CAD build for the part. Positions are in the model's coordinates, mm. A direction names the side the tool comes from. Round coordinates to 2 decimals unless told otherwise and drop trailing zeros. Order: outer loops, then holes, each group sorted by start corner. A loop starts at its lowest first (then second) coordinate and runs counter-clockwise, first axis right, second up. Notation, with made-up numbers: (25.25, -20) - (37.25, -20) arc R10 ccw to (37.25, -4) - close; hole circle Ø6 at (-28, 27.5). An arc over 180 degrees is marked (long way). Write item = value, one per line.
from build123d import *

# Parameters (mm, degrees)
SK_YAW_PLATE_W         = 50
SK_YAW_PLATE_H         = 56.5
SK_YAW_PLATE_R         = 1.7
SK_YAW_PLATE_R_2       = 4
YAW_PLATE_DEPTH        = 6
SK_YAW_PILOT_RECESS_R  = 12.15
YAW_PILOT_RECESS_DEPTH = 2.2
SK_ELBOW_PLATE_W       = 60
SK_ELBOW_PLATE_H       = 154
SK_ELBOW_PLATE_R       = 1.7
SK_ELBOW_PLATE_R_2     = 7
ELBOW_PLATE_DEPTH      = 6


with BuildPart() as part:
    # SK_Yaw_Plate → Yaw_Plate (new body)
    with BuildSketch(Plane.XY.offset(-6)):
        with Locations((0, -3.25)):
            Rectangle(SK_YAW_PLATE_W, SK_YAW_PLATE_H)
        with Locations((16, 0)):
            Circle(SK_YAW_PLATE_R, mode=Mode.SUBTRACT)
        with Locations((8, 13.856406461)):
            Circle(SK_YAW_PLATE_R, mode=Mode.SUBTRACT)
        with Locations((-8, 13.856406461)):
            Circle(SK_YAW_PLATE_R, mode=Mode.SUBTRACT)
        with Locations((-16, 0)):
            Circle(SK_YAW_PLATE_R, mode=Mode.SUBTRACT)
        with Locations((-8, -13.856406461)):
            Circle(SK_YAW_PLATE_R, mode=Mode.SUBTRACT)
        with Locations((8, -13.856406461)):
            Circle(SK_YAW_PLATE_R, mode=Mode.SUBTRACT)
        Circle(SK_YAW_PLATE_R_2, mode=Mode.SUBTRACT)
    extrude(amount=YAW_PLATE_DEPTH)

    # SK_Yaw_Pilot_Recess → Yaw_Pilot_Recess (cut)
    with BuildSketch(Plane.XY):
        Circle(SK_YAW_PILOT_RECESS_R)
    extrude(amount=-YAW_PILOT_RECESS_DEPTH, mode=Mode.SUBTRACT)

    # SK_Elbow_Plate → Elbow_Plate (add)
    with BuildSketch(Plane(origin=(0, -31.5, 0), x_dir=(1, 0, 0), z_dir=(0, 1, 0))):
        with Locations((0, 83)):
            Rectangle(SK_ELBOW_PLATE_W, SK_ELBOW_PLATE_H)
        with Locations(Location((16.263455967, 146.263455967, 0), (0, 0, 270))):
            Circle(SK_ELBOW_PLATE_R, mode=Mode.SUBTRACT)
        with Locations(Location((-16.263455967, 146.263455967, 0), (0, 0, 270))):
            Circle(SK_ELBOW_PLATE_R, mode=Mode.SUBTRACT)
        with Locations(Location((-16.263455967, 113.736544033, 0), (0, 0, 270))):
            Circle(SK_ELBOW_PLATE_R, mode=Mode.SUBTRACT)
        with Locations(Location((16.263455967, 113.736544033, 0), (0, 0, 270))):
            Circle(SK_ELBOW_PLATE_R, mode=Mode.SUBTRACT)
        with Locations(Location((0, 130, 0), (0, 0, 270))):
            Circle(SK_ELBOW_PLATE_R_2, mode=Mode.SUBTRACT)
    extrude(amount=ELBOW_PLATE_DEPTH)


solid = part.part
(1) Probe line 1 along Y through (x, z) = (-8, -3.3); line 2 along Y through (x, z) = (-8, -1.8); line 3 along Y through (x, z) = (0, -1). List the from-to ranges inside material, lowest first.
Solved:
line_1 = -31.5 to -15.56, -12.16 to 12.16, 15.56 to 25
line_2 = -31.5 to -15.56, -12.16 to -9.14, 9.14 to 12.16, 15.56 to 25
line_3 = -31.5 to -12.15, 12.15 to 25
(2) Band-saw the part on D-D on z = -113.5. List the corners of the cut face in (x, y).
Solved:
outline = (-30, -31.5) - (-17.95, -31.5) - (-17.95, -25.5) - (-30, -25.5) - close; (-14.58, -31.5) - (14.58, -31.5) - (14.58, -25.5) - (-14.58, -25.5) - close; (17.95, -31.5) - (30, -31.5) - (30, -25.5) - (17.95, -25.5) - close
(3) Band-saw the part on A-A on y = 0. List the corners of the cut face in (x, z), plus the area to 3 significant figures.
Solved:
outline = (-25, -6) - (-17.7, -6) - (-17.7, 0) - (-25, 0) - close; (-14.3, -6) - (-4, -6) - (-4, -2.2) - (-12.15, -2.2) - (-12.15, 0) - (-14.3, 0) - close; (4, -6) - (14.3, -6) - (14.3, 0) - (12.15, 0) - (12.15, -2.2) - (4, -2.2) - close; (17.7, -6) - (25, -6) - (25, 0) - (17.7, 0) - close
area = 175 mm²
(4) Band-saw the part on B-B on z = -130. List the corners of the cut face in (x, y).
Solved:
outline = (-30, -31.5) - (-7, -31.5) - (-7, -25.5) - (-30, -25.5) - close; (7, -31.5) - (30, -31.5) - (30, -25.5) - (7, -25.5) - close
(5) Drop flat-ended pins along their axis: pin 1 (8 mm diameter, centred on x = -2, z = -42, fed in from +Y); pin 2 (1.5 mm diameter, centred on x = 26.5, y = -28, fed in from +Z); pin 3 (1.8 mm diameter, centred on y = -17, z = -4.5, fed in from -X). Give the stop position or say it passes through.
Solved:
pin_1 = -25.5
pin_2 = -6
pin_3 = -25
(6) Pull direction Y, two halves, no side cores. Call faces 1 (the flat face through (30, -29, -82)), 2 (the flat face through (0, 25, -3)), 3 (the cylindrical face through (-9.7, 13.9, -3)): released by +Y, released by -Y, zero draft, split by the parting line, or undercut.
Solved:
face_1 = zero draft
face_2 = released by +Y
face_3 = undercut
(7) Band-saw the part on C-C on x = -1.5. List the corners of the cut face in (y, z), plus the area to 3 significant figures.
Solved:
outline = (-31.5, -160) - (-25.5, -160) - (-25.5, -136.84) - (-31.5, -136.84) - close; (-31.5, -123.16) - (-25.5, -123.16) - (-25.5, -6) - (-3.71, -6) - (-3.71, -2.2) - (-12.06, -2.2) - (-12.06, 0) - (-31.5, 0) - close; (3.71, -6) - (25, -6) - (25, 0) - (12.06, 0) - (12.06, -2.2) - (3.71, -2.2) - close
area = 1,100 mm²
(8) Tool access for faces 4 (the flat face through (0, -25.5, -84)), 5 (the cylindrical face through (-8.22, -12.17, -3.04)), 6 (the flat face through (27, -29, -6)), 7 (the cylindrical face through (16.338, -28.542, -115.435)), 8 (the cylindrical face through (-2.63, -11.86, -1.08)): list every direction of +Z, -Z, +X, -X, +Y, -Y with a clear straight run to the whole face (end or side of a thin tool).
Solved:
face_4 = -Z, +X, -X, +Y
face_5 = +Z, -Z
face_6 = +Z, +X, +Y, -Y
face_7 = +Y, -Y
face_8 = +Z
